from build123d import *
from OCP.BRepAlgoAPI import BRepAlgoAPI_Cut
from OCP.TopTools import TopTools_ListOfShape

# Parameters (mm, degrees)
BOSS_EXTRUDE1_DEPTH     = 23
CUT_EXTRUDE1_DEPTH      = 120.419428905
CUT_EXTRUDE1_DEPTH_BACK = 120.419428905
SKETCH2_R               = 6
CUT_EXTRUDE4_START      = -28.953391
SKETCH2_3_R             = 4
CUT_EXTRUDE4_DEPTH      = 8


with BuildPart() as part:
    # Sketch1 → Boss-Extrude1 (new, symmetric)
    with BuildSketch(Plane.XY):
        with BuildLine():
            ThreePointArc((-4.105081288, -23.646316999), (-18.364666495, -15.451181979), (-24, 0))
            Line((-24, 0), (-28, 0))
            Line((-28, 0), (-28, 16))
            Line((-28, 16), (-54, 16))
            Line((-54, 16), (-54, -32))
            ThreePointArc((-54, -32), (-56.343145751, -37.656854249), (-62, -40))
            Line((-62, -40), (-99.985564599, -40))
            Line((-99.985564599, -40), (-104, -54))
            Line((-104, -54), (-97.5, -54))
            Line((-97.5, -54), (-97.5, -52))
            Line((-97.5, -52), (-59.034606353, -52))
            Line((-59.034606353, -52), (-54, -52))
            Line((-54, -52), (-54, -42))
            Line((-54, -42), (-26, -42))
            Line((-26, -42), (-26, -52))
            Line((-26, -52), (26, -52))
            Line((26, -52), (26, -42))
            Line((26, -42), (54, -42))
            Line((54, -42), (54, -52))
            Line((54, -52), (97.5, -52))
            Line((97.5, -52), (97.5, -54))
            Line((97.5, -54), (104, -54))
            Line((104, -54), (99.985564599, -40))
            Line((99.985564599, -40), (62, -40))
            ThreePointArc((62, -40), (56.343145751, -37.656854249), (54, -32))
            Line((54, -32), (54, 16))
            Line((54, 16), (28, 16))
            Line((28, 16), (28, 0))
            Line((28, 0), (24, 0))
            ThreePointArc((24, 0), (18.364666495, -15.451181979), (4.105081288, -23.646316999))
            Line((4.105081288, -23.646316999), (4.105081288, -28.953390601))
            Line((4.105081288, -28.953390601), (-4.105081288, -28.953390601))
            Line((-4.105081288, -28.953390601), (-4.105081288, -23.646316999))
        make_face()
    extrude(amount=BOSS_EXTRUDE1_DEPTH, both=True)

    # Sketch2 → Cut-Extrude1 (cut, two sides: drawn at the far end of the back side and taken through both)
    with BuildSketch(Plane(origin=(0, 0, 0), x_dir=(1, 0, 0), z_dir=(0, 1, 0)).offset(-CUT_EXTRUDE1_DEPTH_BACK)):
        with BuildLine():
            Line((-81, -7), (-73, -7))
            ThreePointArc((-73, -7), (-66, 0), (-73, 7))
            Line((-73, 7), (-81, 7))
            ThreePointArc((-81, 7), (-88, 0), (-81, -7))
        make_face()
        with BuildLine():
            ThreePointArc((73, -7), (66, 0), (73, 7))
            Line((73, 7), (81, 7))
            ThreePointArc((81, 7), (88, 0), (81, -7))
            Line((81, -7), (73, -7))
        make_face()
        with Locations(Location((44, 0, 0), (0, 0, 270))):
            Circle(SKETCH2_R)
        with Locations(Location((-44, 0, 0), (0, 0, 270))):
            Circle(SKETCH2_R)
    extrude(amount=CUT_EXTRUDE1_DEPTH + CUT_EXTRUDE1_DEPTH_BACK, mode=Mode.SUBTRACT)


with BuildPart() as cut_extrude4_tool:
    # Sketch2<3> → Cut-Extrude4 (new body)
    with BuildSketch(Plane(origin=(0, 0, 0), x_dir=(1, 0, 0), z_dir=(0, 1, 0)).offset(CUT_EXTRUDE4_START)):
        with Locations(Location((0, 0, 0), (0, 0, 270))):
            Circle(SKETCH2_3_R)
    extrude(amount=-CUT_EXTRUDE4_DEPTH)


with BuildPart() as part_1:
    add(part.part)

    # Cut-Extrude4: cut by cut_extrude4_tool, with a tolerance
    cut_extrude4_stock = TopTools_ListOfShape()
    cut_extrude4_stock.Append(part_1.part.wrapped)
    cut_extrude4_tools = TopTools_ListOfShape()
    cut_extrude4_tools.Append(cut_extrude4_tool.part.wrapped)
    cut_extrude4_cut = BRepAlgoAPI_Cut()
    cut_extrude4_cut.SetArguments(cut_extrude4_stock)
    cut_extrude4_cut.SetTools(cut_extrude4_tools)
    cut_extrude4_cut.SetFuzzyValue(0.00001)
    cut_extrude4_cut.Build()
    add(Compound.cast(cut_extrude4_cut.Shape()).solids(), mode=Mode.REPLACE)


solid = part_1.part
CAD build for the part. Positions are in the model's coordinates, mm. A direction names the side the tool comes from. Coordinates: 2 decimals unless noted, no trailing zeros. Write each loop counter-clockwise with the first axis right and the second up, starting at its lowest first coordinate (ties: lowest second). Pieces come first, ordered by that corner, then holes. Notation, with made-up numbers: M 20.25,64 L 39.25,64 A18 cw 39.25,90 Z; hole C 59,40 d6. An arc over 180 degrees is marked long. Return JSON: item names as keys, results as strings.
Item 1: Slice it at D-D, the plane y = -17.5. Write the cut outline in (x, z), and give its area (3 significant figures).
Findings below:
{"outline": "M -54,-23 L -16.42,-23 L -16.42,23 L -54,23 Z; M 16.42,-23 L 54,-23 L 54,23 L 16.42,23 Z; hole C -44,0 d12; hole C 44,0 d12", "area": "3,230 mm2"}
Item 2: Probe line 1 (X direction, y = -32.5, z = 0); line 2 (X direction, y = -24.5, z = 0); line 3 (X direction, y = -25.5, z = -17.5). List the from-to ranges inside material, lowest first. Write a range as from..to.
Findings below:
{"line 1": "x = -54.02..-50, -38..-4, 4..38, 50..54.02", "line 2": "x = -54..-50, -38..-4.11, 4.11..38, 50..54", "line 3": "x = -54..-4.11, 4.11..54"}
Item 3: Slice it at A-A, the plane y = 4.5. Write the cut outline in (x, z), and give its area (3 significant figures).
Findings below:
{"outline": "M -54,-23 L -28,-23 L -28,23 L -54,23 Z; M 28,-23 L 54,-23 L 54,23 L 28,23 Z; hole C -44,0 d12; hole C 44,0 d12", "area": "2,170 mm2"}
Item 4: Slice it at B-B, the plane x = 44. Write the cut outline in (y, z), and give its area (3 significant figures).
Findings below:
{"outline": "M -42,-23 L 16,-23 L 16,-6 L -42,-6 Z; M -42,6 L 16,6 L 16,23 L -42,23 Z", "area": "1,970 mm2"}
Item 5: Drop flat-ended pins along their axis: pin 1 Ø8.5 at (x, z) = (-45.5, -4.5) entering from -Y; pin 2 Ø19 at (x, z) = (81, 2.5) entering from +Y; pin 3 Ø5 at (y, z) = (-46, 6) entering from +X. Give the stop position or say it passes through.
Findings below:
{"pin 1": "stops at y = -42", "pin 2": "stops at y = -40", "pin 3": "stops at x = 102.42"}
Item 6: Two-plate mould, pull along Z, no slides. Class faces 4 (the flat face through (77, -46, -7)), 5 (the flat face through (-1, -34, 23)), 6 (the flat face through (-101.965, -46.902, 0.322)): +Z half, -Z half, draft (parallel to the pull), parting line (faces both ways), or undercut.
Findings below:
{"face 4": "undercut", "face 5": "+Z half", "face 6": "draft"}
Item 7: Which spindle directions (+Z, -Z, +X, -X, +Y, -Y) get a long thin tool onto all of the face, cutting with end or side? Do faces 1 (the flat face through (65.8, -52, 0.3)), 2 (the flat face through (28, 8, 0)), 3 (the flat face through (35, 16, 0)). Say none if no direction does.
Findings below:
{"face 1": "+Z, -Z, -Y", "face 2": "+Z, -Z, +Y", "face 3": "+Z, -Z, +X, -X, +Y"}
